Could you check a few things on this model? Use its own coordinates, in mm. A direction names the side the tool comes from. Give positions to 0.01 mm unless a question says otherwise; leave off trailing zeros. Write each loop counter-clockwise with the first axis right and the second up, starting at its lowest first coordinate (ties: lowest second). Pieces come first, ordered by that corner, then holes. Notation, with made-up numbers: (55.25, -22) -> (81.25, -22) arc R23 cw to (81.25, 11) -> close; hole circle Ø10 at (3, 48). An arc over 180 degrees is marked (long way). One line per question, with ' | ' between items.
from build123d import *

# Parameters (mm, degrees)
F1_DEPTH = 12.7


with BuildPart() as f1:
    # F0 (on Top) → F1 (new body)
    with BuildSketch(Plane.XY):
        Polygon((219.786288, 270.0056), (-120.990471, -34.7944), (412.409529, -34.7944), (359.51203, 270.0056), align=None)
        with BuildLine():
            ThreePointArc((-54.492408, -22.0944), (-66.356397, -13.92604), (-62.959075, 0.071621))
            Line((-62.959075, 0.071621), (62.597587, 112.372913))
            ThreePointArc((62.597587, 112.372913), (71.770904, 115.587217), (80.530275, 111.373559))
            Line((80.530275, 111.373559), (180.975604, -0.927733))
            ThreePointArc((180.975604, -0.927733), (183.103044, -14.579153), (171.509583, -22.0944))
            Line((171.509583, -22.0944), (-54.492408, -22.0944))
        make_face(mode=Mode.SUBTRACT)
        with BuildLine():
            ThreePointArc((213.436288, 15.079148), (205.267929, 3.215159), (191.270267, 6.612481))
            Line((191.270267, 6.612481), (89.996295, 119.840225))
            ThreePointArc((89.996295, 119.840225), (86.781991, 129.013542), (90.995649, 137.772912))
            Line((90.995649, 137.772912), (192.269622, 228.355107))
            ThreePointArc((192.269622, 228.355107), (205.921042, 230.482547), (213.436288, 218.889086))
            Line((213.436288, 218.889086), (213.436288, 15.079148))
        make_face(mode=Mode.SUBTRACT)
        with BuildLine():
            ThreePointArc((335.022059, 201.344663), (348.200544, 208.646823), (359.079772, 198.223945))
            Line((359.079772, 198.223945), (394.734689, -7.222798))
            ThreePointArc((394.734689, -7.222798), (391.939481, -17.570911), (382.22173, -22.0944))
            Line((382.22173, -22.0944), (252.386372, -22.0944))
            ThreePointArc((252.386372, -22.0944), (241.697535, -16.252881), (240.841618, -4.102079))
            Line((240.841618, -4.102079), (335.022059, 201.344663))
        make_face(mode=Mode.SUBTRACT)
        with BuildLine():
            ThreePointArc((226.13628, 244.6056), (229.856024, 253.585856), (238.83628, 257.3056))
            Line((238.83628, 257.3056), (336.808323, 257.3056))
            ThreePointArc((336.808323, 257.3056), (342.152742, 254.384841), (342.5807, 248.30944))
            Line((342.5807, 248.30944), (238.258657, 20.739642))
            ThreePointArc((238.258657, 20.739642), (231.132045, 17.181889), (226.13628, 23.385803))
            Line((226.13628, 23.385803), (226.13628, 244.6056))
        make_face(mode=Mode.SUBTRACT)
    extrude(amount=F1_DEPTH)


solid = f1.part
Q1. Imagine slicing it at B-B on z = 9.25. Please give me the cut outline in (x, y).
Answer below:
outline: (-120.99, -34.79) -> (412.41, -34.79) -> (359.51, 270.01) -> (219.79, 270.01) -> close; hole (-62.96, 0.07) arc R12.7 ccw to (-54.49, -22.09) -> (171.51, -22.09) arc R12.7 ccw to (180.98, -0.93) -> (80.53, 111.37) arc R12.7 ccw to (62.6, 112.37) -> close; hole (90, 119.84) -> (191.27, 6.61) arc R12.7 ccw to (213.44, 15.08) -> (213.44, 218.89) arc R12.7 ccw to (192.27, 228.36) -> (91, 137.77) arc R12.7 ccw to start; hole (226.14, 23.39) arc R6.35 ccw to (238.26, 20.74) -> (342.58, 248.31) arc R6.35 ccw to (336.81, 257.31) -> (238.84, 257.31) arc R12.7 ccw to (226.14, 244.61) -> close; hole (240.84, -4.1) arc R12.7 ccw to (252.39, -22.09) -> (382.22, -22.09) arc R12.7 ccw to (394.73, -7.22) -> (359.08, 198.22) arc R12.7 ccw to (335.02, 201.34) -> close
Q2. If we mould it in two halves opening along Y, with no side actions, what happens to faces 1 (the flat face through (287, 257.306, 6)), 2 (the flat face through (223, 84, 12.7)), 3 (the flat face through (142, -34.794, 6)), 4 (the cylindrical face through (71.631, 115.594, 6.261))? For each: +Y half, -Y half, draft (parallel to the pull), parting line (faces both ways), or undercut.
Answer below:
face 1: undercut | face 2: draft | face 3: -Y half | face 4: undercut
Q3. On a 3-axis mill with a long thin cutter (end or side, diameter ignored), from which of +Z, -Z, +X, -X, +Y, -Y can I reach the whole of each face in a straight line? I mean faces 5 (the cylindrical face through (392, -17.5, 6.3)), 6 (the flat face through (386.33, 115.47, 6.26)). Say none if no direction works.
Answer below:
face 5: +Z, -Z | face 6: +Z, -Z, +X, +Y
Q4. If I drill on line 1 along X through (y, z) = (136, 6.25); line 2 along X through (y, z) = (10, 11); line 3 along Y through (x, z) = (88.5, 1.75), over which ranges is the centre line in solid material (lowest first)?
Answer below:
line 1: x = 69.96 to 89.36, 213.44 to 226.14, 291.1 to 305.07, 369.88 to 382.77 | line 2: x = -70.91 to -51.86, 171.2 to 188.24, 212.38 to 247.31, 391.75 to 404.64 | line 3: y = -34.79 to -22.09, 102.46 to 121.89, 134.72 to 152.58
Q5. Will these pins go through, and if not, where does the flat tip stop? pin 1 (1 mm diameter, centred on y = 152, z = 5, fed in from -X); pin 2 (4 mm diameter, centred on y = 149, z = 7.5, fed in from -X); pin 3 (4 mm diameter, centred on x = 132.5, z = 4.5, fed in from +Y).
Answer below:
pin 1: stops at x = 87.29 | pin 2: stops at x = 82.26 | pin 3: stops at y = 193.72
Q6. Imagine slicing it at D-D on y = 175. Please give me the cut outline in (x, z), and give its area (3 significant figures).
Answer below:
outline: (113.57, 0) -> (132.62, 0) -> (132.62, 12.7) -> (113.57, 12.7) -> close; (213.44, 0) -> (226.14, 0) -> (226.14, 12.7) -> (213.44, 12.7) -> close; (308.97, 0) -> (322.95, 0) -> (322.95, 12.7) -> (308.97, 12.7) -> close; (363.11, 0) -> (376, 0) -> (376, 12.7) -> (363.11, 12.7) -> close | area: 744 mm^2
Q7. Imagine slicing it at A-A on x = 116. Please give me the cut outline in (y, z), and give its area (3 significant figures).
Answer below:
outline: (-34.79, 0) -> (-22.09, 0) -> (-22.09, 12.7) -> (-34.79, 12.7) -> close; (71.72, 0) -> (90.77, 0) -> (90.77, 12.7) -> (71.72, 12.7) -> close; (160.14, 0) -> (177.18, 0) -> (177.18, 12.7) -> (160.14, 12.7) -> close | area: 620 mm^2
Q8. Imagine slicing it at C-C on y = 29.5. Please give me the cut outline in (x, z), and give its area (3 significant figures).
Answer below:
outline: (-49.11, 0) -> (-30.06, 0) -> (-30.06, 12.7) -> (-49.11, 12.7) -> close; (153.76, 0) -> (170.8, 0) -> (170.8, 12.7) -> (153.76, 12.7) -> close; (213.44, 0) -> (226.14, 0) -> (226.14, 12.7) -> (213.44, 12.7) -> close; (242.27, 0) -> (256.25, 0) -> (256.25, 12.7) -> (242.27, 12.7) -> close; (388.36, 0) -> (401.25, 0) -> (401.25, 12.7) -> (388.36, 12.7) -> close | area: 961 mm^2
